Work out the finished part from the listing and answer in its coordinate system (mm). A direction names the side the tool comes from. Coordinates: 2 decimals unless noted, no trailing zeros. Order: outer loops, then holes, each group sorted by start corner. A loop starts at its lowest first (then second) coordinate and runs counter-clockwise, first axis right, second up.
1. Flat-ended cylindrical pins translate along their axes: pin 1 Ø5.5 at (x, y) = (22, 10) entering from +Z; pin 2 Ø6 at (x, y) = (30, 10) entering from +Z; pin 3 Ø12 at (x, z) = (8.5, 13.5) entering from +Y. Find the tip coordinate at first contact, or state that the pin passes through.
2. Find the intervals of material crossed by probe 1 along X at (y, z) = (0.7, 10); probe 2 along Y at (x, z) = (30, 1.35); probe 3 along X at (y, z) = (12.25, 1.25), in increasing order.
3. The part is cut by section A-A, the plane z = 10. Give the vertices of the cut face in (x, y), then the cut area to 3 significant figures.
4. A tool of negligible diameter and unlimited length cuts with its end or side. For faces 4 (the cylindrical face through (26.827, 0.986, 9.295)), 5 (the flat face through (20, 11, 2)), from which of +Z, -Z, +X, -X, +Y, -Y can it reach the whole face along a straight path? Write none if from no direction.
5. The part is cut by section D-D, the plane x = 22. Give the vertices of the cut face in (y, z), then the cut area to 3 significant figures.
6. The part is cut by section B-B, the plane x = 30. Give the vertices of the cut face in (y, z), then the cut area to 3 significant figures.
7. Determine the mould class of faces 1 (the flat face through (40, 1.8, 6.3)), 2 (the flat face through (0, 1.8, 6.3)), 3 (the cylindrical face through (6.753, 10.143, 0.986)) for opening direction X: +X half, -X half, draft (parallel to the pull), parting line (faces both ways), or undercut.
```python
from build123d import *

# Parameters (mm, degrees)
SKETCH1_W           = 40
SKETCH1_H           = 20
SKETCH1_R           = 3.25
BOSS_EXTRUDE1_DEPTH = 2
SKETCH3_W           = 40
SKETCH3_H           = 20
SKETCH3_R           = 3.25
BOSS_EXTRUDE2_DEPTH = 2


with BuildPart() as part:
    # Sketch1 → Boss-Extrude1 (new body)
    with BuildSketch(Plane.XY):
        with Locations((20, 10)):
            Rectangle(SKETCH1_W, SKETCH1_H)
        with Locations((10, 10)):
            Circle(SKETCH1_R, mode=Mode.SUBTRACT)
        with Locations((30, 10)):
            Circle(SKETCH1_R, mode=Mode.SUBTRACT)
    extrude(amount=BOSS_EXTRUDE1_DEPTH)

    # Sketch3 → Boss-Extrude2 (add)
    with BuildSketch(Plane(origin=(0, 0, 0), x_dir=(1, 0, 0), z_dir=(0, 1, 0))):
        with Locations((20, -10)):
            Rectangle(SKETCH3_W, SKETCH3_H)
        with Locations(Location((10, -10, 0), (0, 0, 270))):
            Circle(SKETCH3_R, mode=Mode.SUBTRACT)
        with Locations(Location((30, -10, 0), (0, 0, 270))):
            Circle(SKETCH3_R, mode=Mode.SUBTRACT)
    extrude(amount=BOSS_EXTRUDE2_DEPTH)


solid = part.part
```
Geometry says:
1. pin 1: stops at z = 2
1. pin 2: passes through
1. pin 3: stops at y = 2
2. probe 1: x = 0 to 6.75, 13.25 to 26.75, 33.25 to 40
2. probe 2: y = 0 to 6.75, 13.25 to 20
2. probe 3: x = 0 to 7.65, 12.35 to 27.65, 32.35 to 40
3. outline: (0, 0) - (6.75, 0) - (6.75, 2) - (0, 2) - close; (13.25, 0) - (26.75, 0) - (26.75, 2) - (13.25, 2) - close; (33.25, 0) - (40, 0) - (40, 2) - (33.25, 2) - close
3. area: 54.0 mm2
4. face 4: +Y, -Y
4. face 5: +Z, +X, -X, +Y
5. outline: (0, 0) - (20, 0) - (20, 2) - (2, 2) - (2, 20) - (0, 20) - close
5. area: 76.0 mm2
6. outline: (0, 0) - (6.75, 0) - (6.75, 2) - (2, 2) - (2, 6.75) - (0, 6.75) - close; (0, 13.25) - (2, 13.25) - (2, 20) - (0, 20) - close; (13.25, 0) - (20, 0) - (20, 2) - (13.25, 2) - close
6. area: 50.0 mm2
7. face 1: +X half
7. face 2: -X half
7. face 3: undercut
